Verification items for the finished model (mm, model axes). Give positions to 0.01 mm unless a question says otherwise; leave off trailing zeros. Order: outer loops, then holes, each group sorted by start corner. A loop starts at its lowest first (then second) coordinate and runs counter-clockwise, first axis right, second up. Notation, with made-up numbers: (59, 33.25) - (76, 33.25) arc R13 cw to (76, 50.25) - close; hole circle Ø10 at (-33, 29.25). An arc over 180 degrees is marked (long way). Answer as a JSON object with one key per item and string values. Group by question number.
(1) Section check C-C (z = 13.5). Count the separate pieces of the cut face and the enclosed holes in it, then the cut area to 3 significant figures.
(2) Section check B-B (y = 0). Record the boundary of the cut face in (x, z).
(3) Section check A-A (x = 14.75). Record the boundary of the cut face in (y, z), then the cut area to 3 significant figures.
(4) Thickness scan on line 1 (Y direction, x = 0.25, z = 58.5); line 2 (X direction, y = 2.5, z = 94.5); line 3 (X direction, y = 12.5, z = 11). Record the ranges inside material, lowest first.
(5) Section check D-D (x = -7). Record the boundary of the cut face in (y, z), then the cut area to 3 significant figures.
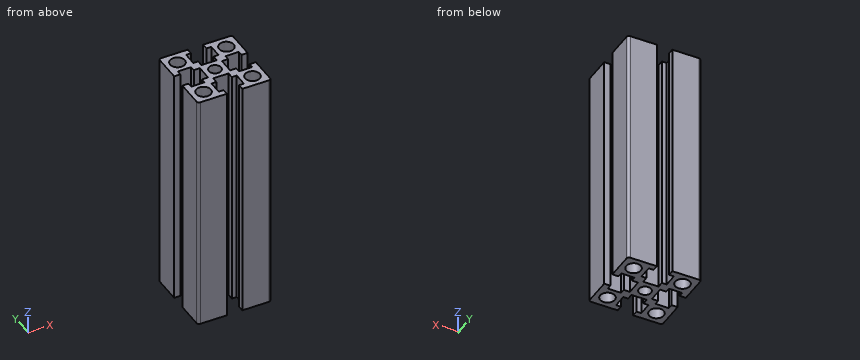
```python
from build123d import *

# Parameters (mm, degrees)
SKETCH_1_R      = 3
SKETCH_1_R_2    = 2.5
EXTRUDE_1_DEPTH = 100


with BuildPart() as part:
    # 草图1 → 凸台-拉伸1 (new body)
    with BuildSketch(Plane.XY):
        with BuildLine():
            Line((-11.436512183, -15.117205795), (-11.436512183, -4.267205795))
            Line((-11.436512183, -4.267205795), (-8.936512183, -4.267205795))
            Line((-8.936512183, -4.267205795), (-8.936512183, -6.267205795))
            Line((-8.936512183, -6.267205795), (-3.436512183, -6.267205795))
            Line((-3.436512183, -6.267205795), (-3.436512183, -4.267205795))
            Line((-3.436512183, -4.267205795), (-0.936512183, -4.267205795))
            Line((-0.936512183, -4.267205795), (-0.936512183, 2.032794205))
            Line((-0.936512183, 2.032794205), (-3.436512183, 2.032794205))
            Line((-3.436512183, 2.032794205), (-3.436512183, 4.032794205))
            Line((-3.436512183, 4.032794205), (-8.936512183, 4.032794205))
            Line((-8.936512183, 4.032794205), (-8.936512183, 2.032794205))
            Line((-8.936512183, 2.032794205), (-11.436512183, 2.032794205))
            Line((-11.436512183, 2.032794205), (-11.436512183, 12.882794205))
            ThreePointArc((-11.436512183, 12.882794205), (-11.143618964, 13.589900986), (-10.436512183, 13.882794205))
            Line((-10.436512183, 13.882794205), (0.413487817, 13.882794205))
            Line((0.413487817, 13.882794205), (0.413487817, 11.382794205))
            Line((0.413487817, 11.382794205), (-1.586512183, 11.382794205))
            Line((-1.586512183, 11.382794205), (-1.586512183, 5.882794205))
            Line((-1.586512183, 5.882794205), (0.413487817, 5.882794205))
            Line((0.413487817, 5.882794205), (0.413487817, 3.382794205))
            Line((0.413487817, 3.382794205), (6.713487817, 3.382794205))
            Line((6.713487817, 3.382794205), (6.713487817, 5.882794205))
            Line((6.713487817, 5.882794205), (8.713487817, 5.882794205))
            Line((8.713487817, 5.882794205), (8.713487817, 11.382794205))
            Line((8.713487817, 11.382794205), (6.713487817, 11.382794205))
            Line((6.713487817, 11.382794205), (6.713487817, 13.882794205))
            Line((6.713487817, 13.882794205), (17.563487817, 13.882794205))
            ThreePointArc((17.563487817, 13.882794205), (18.270594598, 13.589900986), (18.563487817, 12.882794205))
            Line((18.563487817, 12.882794205), (18.563487817, 2.032794205))
            Line((18.563487817, 2.032794205), (16.063487817, 2.032794205))
            Line((16.063487817, 2.032794205), (16.063487817, 4.032794205))
            Line((16.063487817, 4.032794205), (10.563487817, 4.032794205))
            Line((10.563487817, 4.032794205), (10.563487817, 2.032794205))
            Line((10.563487817, 2.032794205), (8.063487817, 2.032794205))
            Line((8.063487817, 2.032794205), (8.063487817, -4.267205795))
            Line((8.063487817, -4.267205795), (10.563487817, -4.267205795))
            Line((10.563487817, -4.267205795), (10.563487817, -6.267205795))
            Line((10.563487817, -6.267205795), (16.063487817, -6.267205795))
            Line((16.063487817, -6.267205795), (16.063487817, -4.267205795))
            Line((16.063487817, -4.267205795), (18.563487817, -4.267205795))
            Line((18.563487817, -4.267205795), (18.563487817, -15.117205795))
            ThreePointArc((18.563487817, -15.117205795), (18.270594598, -15.824312576), (17.563487817, -16.117205795))
            Line((17.563487817, -16.117205795), (6.713487817, -16.117205795))
            Line((6.713487817, -16.117205795), (6.713487817, -13.617205795))
            Line((6.713487817, -13.617205795), (8.713487817, -13.617205795))
            Line((8.713487817, -13.617205795), (8.713487817, -8.117205795))
            Line((8.713487817, -8.117205795), (6.713487817, -8.117205795))
            Line((6.713487817, -8.117205795), (6.713487817, -5.617205795))
            Line((6.713487817, -5.617205795), (0.413487817, -5.617205795))
            Line((0.413487817, -5.617205795), (0.413487817, -8.117205795))
            Line((0.413487817, -8.117205795), (-1.586512183, -8.117205795))
            Line((-1.586512183, -8.117205795), (-1.586512183, -13.617205795))
            Line((-1.586512183, -13.617205795), (0.413487817, -13.617205795))
            Line((0.413487817, -13.617205795), (0.413487817, -16.117205795))
            Line((0.413487817, -16.117205795), (-10.436512183, -16.117205795))
            ThreePointArc((-10.436512183, -16.117205795), (-11.143618964, -15.824312576), (-11.436512183, -15.117205795))
        make_face()
        with Locations((-6.436512183, 8.882794205)):
            Circle(SKETCH_1_R, mode=Mode.SUBTRACT)
        with Locations((-6.436512183, -11.117205795)):
            Circle(SKETCH_1_R, mode=Mode.SUBTRACT)
        with Locations((13.563487817, -11.117205795)):
            Circle(SKETCH_1_R, mode=Mode.SUBTRACT)
        with Locations((13.563487817, 8.882794205)):
            Circle(SKETCH_1_R, mode=Mode.SUBTRACT)
        with Locations((3.563487817, -1.117205795)):
            Circle(SKETCH_1_R_2, mode=Mode.SUBTRACT)
    extrude(amount=EXTRUDE_1_DEPTH)


solid = part.part
```
Solutions:
{
 "1": {"separate pieces": "1", "enclosed holes": "5", "area": "414 mm2"},
 "2": {"outline": "(-0.94, 0) - (1.33, 0) - (1.33, 100) - (-0.94, 100) - close; (5.8, 0) - (8.06, 0) - (8.06, 100) - (5.8, 100) - close"},
 "3": {"outline": "(-16.12, 0) - (-13.87, 0) - (-13.87, 100) - (-16.12, 100) - close; (-8.36, 0) - (-6.27, 0) - (-6.27, 100) - (-8.36, 100) - close; (4.03, 0) - (6.13, 0) - (6.13, 100) - (4.03, 100) - close; (11.64, 0) - (13.88, 0) - (13.88, 100) - (11.64, 100) - close", "area": "868 mm2"},
 "4": {"line 1": "y = -16.12 to -13.62, -8.12 to 5.88, 11.38 to 13.88", "line 2": "x = -11.44 to -8.94, -3.44 to 10.56, 16.06 to 18.56", "line 3": "x = -11.44 to 0.41, 6.71 to 18.56"},
 "5": {"outline": "(-16.12, 0) - (-14.06, 0) - (-14.06, 100) - (-16.12, 100) - close; (-8.17, 0) - (-6.27, 0) - (-6.27, 100) - (-8.17, 100) - close; (4.03, 0) - (5.94, 0) - (5.94, 100) - (4.03, 100) - close; (11.83, 0) - (13.88, 0) - (13.88, 100) - (11.83, 100) - close", "area": "791 mm2"}
}
